Work out the finished part from the listing and answer in its coordinate system (mm). A direction names the side the tool comes from. Round coordinates to 2 decimals unless told otherwise and drop trailing zeros. Write each loop counter-clockwise with the first axis right and the second up, starting at its lowest first coordinate (ties: lowest second). Pieces come first, ordered by that corner, then holes.
1. A tool of negligible diameter and unlimited length cuts with its end or side. For faces 5 (the face through (0, 21, -10)), 6 (the face through (24, 34.5, 0)), 7 (the face through (20, 16, 0)), 8 (the face through (-20, 39, 0)), 9 (the face through (-20, 16, 0)), from which of +Z, -Z, +X, -X, +Y, -Y can it reach the whole face along a straight path? Write none if from no direction.
2. Straight lines are drawn through the part: probe 1 along Z at (x, y) = (24, 32.7); probe 2 along X at (y, z) = (34, 5); probe 3 along X at (y, z) = (18.5, 4.25). For each, find the intervals that lie inside material, in ascending order.
3. Find section B-B (z = -5). Write down the section's boundary in (x, y), and give its area (4 significant figures).
4. Flat-ended cylindrical pins translate along their axes: pin 1 Ø5 at (x, z) = (-24, -5) entering from -Y; pin 2 Ø4 at (y, z) = (40.5, 3) entering from +X; pin 3 Ø1.5 at (x, z) = (-3, -0.5) entering from +Y. Find the tip coordinate at first contact, or state that the pin passes through.
5. Find section D-D (x = -9.86). Write down the section's boundary in (y, z).
6. Find section A-A (x = 24). Write down the section's boundary in (y, z).
7. Find section C-C (z = -8). Write down the section's boundary in (x, y), and give its area (3 significant figures).
8. Determine the mould class of faces 1 (the face through (-12.241, 45.159, -1.825)), 2 (the face through (-24, 32, 0)), 3 (the face through (27.5, 33, 0)), 4 (the face through (26.146, 33.268, -5.676)) for opening direction X: pulls with the +X half, pulls with the -X half, needs draft (parallel to the pull), parting line crosses it, or undercut.
Autodesk Inventor part; units mm, degrees
ref_plane "YZ Plane" through (0, 0, 0) normal (1, 0, 0) x (0, 1, 0)
ref_plane "XZ Plane" through (0, 0, 0) normal (0, 1, 0) x (-1, 0, 0)
ref_plane "XY Plane" through (0, 0, 0) normal (0, 0, 1) x (1, 0, 0)
sketch "Sketch1" plane through (0, 0, 0) normal (0, 1, 0) x (-1, 0, 0)
  line L0 (-20, 10) -> (20, 10)
  line L1 (20, 10) -> (20, -10)
  line L2 (20, -10) -> (-20, -10)
  line L3 (-20, -10) -> (-20, 10)
  line L4 (-20, 10) -> (20, -10) construction
  line L5 (20, 10) -> (-20, -10) construction
  point P0 (0, 0)
  dimension "d0" = 40
  dimension "d1" = 20
extrude "Extrusion1" add sketch "Sketch1" along normal blind 43
sketch "Sketch2" plane through (-20, 0, 10) normal (0, 0, 1) x (1, 0, 0)
  line L0 (-7.5, 34.5) -> (47.5, 34.5)
  line L1 (47.5, 34.5) -> (47.5, 32)
  line L2 (47.5, 32) -> (-7.5, 32)
  line L3 (-7.5, 32) -> (-7.5, 34.5)
  line L4 (0, 0) -> (40, 0)
  line L5 (0, 0) -> (0, 43)
  point P0 (20, 0)
  point P1 (-7.5, 33.25)
  dimension "d4" = 55
  dimension "d5" = 2.5
  dimension "d6" = 32
  dimension "d7" = 7.5
extrude "Extrusion2" add sketch "Sketch2" against normal up to surface (20 mm away)
sketch "Sketch3" plane through (-27.5, 34.5, 10) normal (0, 1, 0) x (1, 0, 0)
  line L0 (0, 0) -> (0, 20)
  line L1 (0, 10) -> (55, 10) construction
  line L2 (55, 0) -> (55, 20)
  line L3 (7.5, 0) -> (47.5, 0)
  line L4 (27.5, 0) -> (27.5, 20) construction
  line L5 (47.5, 20) -> (7.5, 20)
  circle A0 centre (3.5, 5) radius 2.25
  circle A1 centre (3.5, 15) radius 2.25
  circle A2 centre (51.5, 5) radius 2.25
  circle A3 centre (51.5, 15) radius 2.25
  point P0 (27.5, 10)
  dimension "d10" = 4.5
  dimension "d11" = 5
  dimension "d12" = 24
extrude "Extrusion3" cut sketch "Sketch3" against normal through all
sketch "Sketch4" plane through (0, 43, 0) normal (0, 1, 0) x (1, 0, 0)
  line L0 (-27.5, -10) -> (-27.5, 10)
  line L1 (-27.5, 0) -> (27.5, 0) construction
  line L2 (27.5, -10) -> (27.5, 10)
  line L3 (0, -10) -> (0, 10) construction
  line L4 (20, 10) -> (-20, 10)
  circle A0 centre (-9.86, 0) radius 3
  point P0 (0, 0)
  dimension "d15" = 6
  dimension "d16" = 9.86
extrude "Extrusion4" add sketch "Sketch4" along normal blind 4.38
properties part number "feetech_25kg_servo" material "Acetal Resin, Black"
Worked answers:
1. face 5: -Z, +X, -X, +Y, -Y
1. face 6: +Z, -Z, +X, +Y
1. face 7: +Z, -Z, +X, -Y
1. face 8: +Z, -Z, -X, +Y
1. face 9: +Z, -Z, -X, -Y
2. probe 1: z = -10 to -7.25, -2.75 to 2.75, 7.25 to 10
2. probe 2: x = -27.5 to -26.25, -21.75 to 21.75, 26.25 to 27.5
2. probe 3: x = -20 to 20
3. outline: (-27.5, 32) - (-26.25, 32) - (-26.25, 34.5) - (-27.5, 34.5) - close; (-21.75, 32) - (-20, 32) - (-20, 0) - (20, 0) - (20, 32) - (21.75, 32) - (21.75, 34.5) - (20, 34.5) - (20, 43) - (-20, 43) - (-20, 34.5) - (-21.75, 34.5) - close; (26.25, 32) - (27.5, 32) - (27.5, 34.5) - (26.25, 34.5) - close
3. area: 1,735 mm2
4. pin 1: stops at y = 32
4. pin 2: stops at x = 20
4. pin 3: stops at y = 43
5. outline: (0, -10) - (43, -10) - (43, -3) - (47.38, -3) - (47.38, 3) - (43, 3) - (43, 10) - (0, 10) - close
6. outline: (32, -10) - (34.5, -10) - (34.5, -7.25) - (32, -7.25) - close; (32, -2.75) - (34.5, -2.75) - (34.5, 2.75) - (32, 2.75) - close; (32, 7.25) - (34.5, 7.25) - (34.5, 10) - (32, 10) - close
7. outline: (-27.5, 32) - (-20, 32) - (-20, 0) - (20, 0) - (20, 32) - (27.5, 32) - (27.5, 34.5) - (20, 34.5) - (20, 43) - (-20, 43) - (-20, 34.5) - (-27.5, 34.5) - close
7. area: 1,760 mm2
8. face 1: parting line crosses it
8. face 2: needs draft
8. face 3: pulls with the +X half
8. face 4: undercut
